Input: part model. Units: mm. Frame: model coordinates. Face numbers are marked on the shaded views. A direction names the side the tool comes from. Give positions to 0.01 mm unless a question says otherwise; leave off trailing zeros. Order: outer loops, then holes, each group sorted by start corner. A loop starts at its lowest first (then second) coordinate and runs counter-clockwise, first axis right, second up. Notation, with made-up numbers: (64, 7.5) - (116, 7.5) arc R15 cw to (116, 36.5) - close; hole circle Ø4 at (29.25, 61). An arc over 180 degrees is marked (long way). Use a Markdown table: item, result.
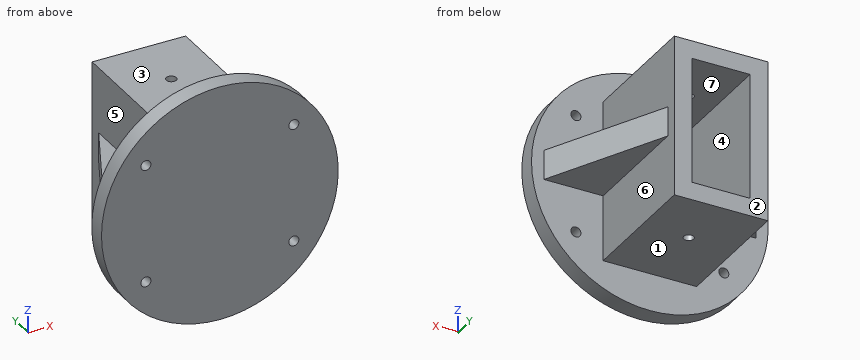
from build123d import *

# Parameters (mm, degrees)
CROQUIS1_W              = 31.6
CROQUIS1_H              = 54.6
CROQUIS1_W_2            = 19.6
CROQUIS1_H_2            = 42.6
SALIENTE_EXTRUIR1_DEPTH = 50
CROQUIS2_R              = 40
SALIENTE_EXTRUIR2_DEPTH = 6
NERVIO4_REACH           = 77.498
CROQUIS3_WALL_W         = 197.718048256
CROQUIS3_WALL_H         = 10
CROQUIS4_R              = 1.7
CORTAR_EXTRUIR1_DEPTH   = 10
CROQUIS5_R              = 1.7
CORTAR_EXTRUIR2_DEPTH   = 60


with BuildPart() as part:
    # Croquis1 → Saliente-Extruir1 (new body)
    with BuildSketch(Plane(origin=(0, 0, 0), x_dir=(1, 0, 0), z_dir=(0, 1, 0))):
        Rectangle(CROQUIS1_W, CROQUIS1_H)
        Rectangle(CROQUIS1_W_2, CROQUIS1_H_2, mode=Mode.SUBTRACT)
    extrude(amount=SALIENTE_EXTRUIR1_DEPTH)

    # Croquis2 → Saliente-Extruir2 (add)
    with BuildSketch(Plane(origin=(0, 0, 0), x_dir=(-1, 0, 0), z_dir=(0, -1, 0))):
        with Locations(Location((0, 0, 0), (0, 0, 90))):
            Circle(CROQUIS2_R)
    extrude(amount=-SALIENTE_EXTRUIR2_DEPTH)

    # Croquis3 wall → Nervio4 (add, up to next)
    with BuildSketch(Plane(origin=(-25.8, 26, 0), x_dir=(-0.4472135955, -0.894427191, 0), z_dir=(0.894427191, -0.4472135955, 0)), mode=Mode.PRIVATE) as nervio4_sk1:
        Rectangle(CROQUIS3_WALL_W, CROQUIS3_WALL_H)
    nervio4_tool1 = extrude(nervio4_sk1.sketch, amount=NERVIO4_REACH, mode=Mode.PRIVATE) - part.part
    nervio4 = nervio4_tool1.solids().sort_by_distance((-25.8, 26, 0))[0]
    add(nervio4)

    # Simetría1: Nervio4 across plane
    add(nervio4.mirror(Plane(origin=(0, 0, 0), x_dir=(0, 0, 1), z_dir=(1, 0, 0))))

    # Croquis4 → Cortar-Extruir1 (cut)
    with BuildSketch(Plane(origin=(0, 6, 0), x_dir=(1, 0, 0), z_dir=(0, 1, 0))):
        with Locations(Location((-25, 20, 0), (0, 0, 270))):
            Circle(CROQUIS4_R)
        with Locations(Location((-25, -20, 0), (0, 0, 270))):
            Circle(CROQUIS4_R)
        with Locations(Location((25, -20, 0), (0, 0, 270))):
            Circle(CROQUIS4_R)
        with Locations(Location((25, 20, 0), (0, 0, 270))):
            Circle(CROQUIS4_R)
    extrude(amount=-CORTAR_EXTRUIR1_DEPTH, mode=Mode.SUBTRACT)

    # Croquis5 → Cortar-Extruir2 (cut)
    with BuildSketch(Plane.XY.offset(27.3)):
        with Locations((0, 30)):
            Circle(CROQUIS5_R)
    extrude(amount=-CORTAR_EXTRUIR2_DEPTH, mode=Mode.SUBTRACT)


solid = part.part
1. Mould query, pull axis Z, two halves, no side actions, for the marked faces 1, 2, 3 and 4. Classes: pulls with the +Z half, pulls with the -Z half, needs draft (parallel to the pull), parting line crosses it, or undercut.
Response:
| item | result |
|---|---|
| face 1 | pulls with the -Z half |
| face 2 | needs draft |
| face 3 | pulls with the +Z half |
| face 4 | undercut |
2. Material intervals for line 1 along Y through (x, z) = (0, -23.15); line 2 along X through (y, z) = (47, 11.5); line 3 along Y through (x, z) = (28, -16), sorted ascending.
Response:
| item | result |
|---|---|
| line 1 | y = 0 to 28.3, 31.7 to 50 |
| line 2 | x = -15.8 to -9.8, 9.8 to 15.8 |
| line 3 | y = 0 to 6 |
3. Section query B-B (x = 0). Return loops of the section in (y, z).
Response:
| item | result |
|---|---|
| outline | (0, -40) - (6, -40) - (6, -27.3) - (28.3, -27.3) - (28.3, -21.3) - (6, -21.3) - (6, 21.3) - (28.3, 21.3) - (28.3, 27.3) - (6, 27.3) - (6, 40) - (0, 40) - close; (31.7, -27.3) - (50, -27.3) - (50, -21.3) - (31.7, -21.3) - close; (31.7, 21.3) - (50, 21.3) - (50, 27.3) - (31.7, 27.3) - close |
4. Set-up query: the marked faces 5, 6 and 7. Return all of +Z, -Z, +X, -X, +Y, -Y with unobstructed straight access to the full face (end or side cutting, diameter ignored); none if empty.
Response:
| item | result |
|---|---|
| face 5 | -X, +Y |
| face 6 | +X, +Y |
| face 7 | +Y |
5. Section query A-A (y = 10.5). Return loops of the section in (x, z), then the cut area to 3 significant figures.
Response:
| item | result |
|---|---|
| outline | (-33.55, -5) - (-15.8, -5) - (-15.8, -27.3) - (15.8, -27.3) - (15.8, -5) - (33.55, -5) - (33.55, 5) - (15.8, 5) - (15.8, 27.3) - (-15.8, 27.3) - (-15.8, 5) - (-33.55, 5) - close; hole (-9.8, -21.3) - (9.8, -21.3) - (9.8, 21.3) - (-9.8, 21.3) - close |
| area | 1,250 mm^2 |
6. Section query C-C (z = -20). Return loops of the section in (x, y).
Response:
| item | result |
|---|---|
| outline | (-34.64, 0) - (-26.7, 0) - (-26.7, 6) - (-34.64, 6) - close; (-23.3, 0) - (23.3, 0) - (23.3, 6) - (15.8, 6) - (15.8, 50) - (9.8, 50) - (9.8, 6) - (-9.8, 6) - (-9.8, 50) - (-15.8, 50) - (-15.8, 6) - (-23.3, 6) - close; (26.7, 0) - (34.64, 0) - (34.64, 6) - (26.7, 6) - close |
7. Section query D-D (y = 30). Return loops of the section in (x, z).
Response:
| item | result |
|---|---|
| outline | (-23.8, -5) - (-15.8, -5) - (-15.8, -27.3) - (-1.7, -27.3) - (-1.7, -21.3) - (-9.8, -21.3) - (-9.8, 21.3) - (-1.7, 21.3) - (-1.7, 27.3) - (-15.8, 27.3) - (-15.8, 5) - (-23.8, 5) - close; (1.7, -27.3) - (15.8, -27.3) - (15.8, -5) - (23.8, -5) - (23.8, 5) - (15.8, 5) - (15.8, 27.3) - (1.7, 27.3) - (1.7, 21.3) - (9.8, 21.3) - (9.8, -21.3) - (1.7, -21.3) - close |
8. Pin query (flat end, axial travel): pin 1 (10 mm diameter, centred on x = -2.5, y = 23, fed in from +Z); pin 2 (5 mm diameter, centred on y = 26.5, z = -1, fed in from -X); pin 3 (5.5 mm diameter, centred on x = -25, z = -20, fed in from +Y). Return the tip coordinate at first contact, or that it passes through.
Response:
| item | result |
|---|---|
| pin 1 | stops at z = 27.3 |
| pin 2 | stops at x = -26.8 |
| pin 3 | stops at y = 6 |
